from build123d import *

# Parameters (mm, degrees)
F0_W     = 72
F0_H     = 20
F0_R     = 3
F1_DEPTH = 4.5
F2_R     = 7.5
F2_R_2   = 3
F3_DEPTH = 5.5
F4_SIZE  = 5
F6_D     = 4.2


with BuildPart() as f1:
    # F0 (on Front) → F1 (new body)
    with BuildSketch(Plane.XZ):
        Rectangle(F0_W, F0_H)
        Circle(F0_R, mode=Mode.SUBTRACT)
    extrude(amount=F1_DEPTH)

    # F2 (on face) → F3 (join)
    with BuildSketch(Plane.XZ.offset(4.5)):
        Circle(F2_R)
        Circle(F2_R_2, mode=Mode.SUBTRACT)
    extrude(amount=F3_DEPTH)

    # F4
    f4_edges = [f1.edges().sort_by_distance(p)[0] for p in [
        (36, -2.25, 10),
        (36, -2.25, -10),
        (-36, -2.25, 10),
        (-36, -2.25, -10),
    ]]
    chamfer(f4_edges, length=F4_SIZE)

    # F6 (through all)
    with Locations(Plane(origin=(0, 0, 0), x_dir=(-1, 0, 0), z_dir=(0, 1, 0))):
        with Locations((-30, 0), (30, 0)):
            Hole(F6_D / 2)


solid = f1.part
For this review, take the finished solid that the model builds, in its own axes (mm). A direction names the side the tool comes from. Round coordinates to 2 decimals unless told otherwise and drop trailing zeros. Write each loop counter-clockwise with the first axis right and the second up, starting at its lowest first coordinate (ties: lowest second). Pieces come first, ordered by that corner, then holes. Notation, with made-up numbers: (-25.5, 36) - (-14.5, 36) arc R19 ccw to (-14.5, 43) - close; hole circle Ø3 at (81, 19). An arc over 180 degrees is marked (long way). Use a Markdown table: item, result.
Q1. We need section A-A (x = 30). Give the boundary of the cut face in (y, z), plus the area to 3 significant figures.
Derived:
| item | result |
|---|---|
| outline | (-4.5, -10) - (0, -10) - (0, -2.1) - (-4.5, -2.1) - close; (-4.5, 2.1) - (0, 2.1) - (0, 10) - (-4.5, 10) - close |
| area | 71.1 mm2 |
Q2. We need section C-C (y = -3.75). Give the boundary of the cut face in (x, z).
Derived:
| item | result |
|---|---|
| outline | (-36, -5) - (-31, -10) - (31, -10) - (36, -5) - (36, 5) - (31, 10) - (-31, 10) - (-36, 5) - close; hole circle Ø4.2 at (-30, 0); hole circle Ø6 at (0, 0); hole circle Ø4.2 at (30, 0) |
Q3. Clearance check with flat-ended pins moving along their axes: pin 1 (3 mm diameter, centred on x = 13.5, z = -5, fed in from -Y); pin 2 (3 mm diameter, centred on x = -0.5, z = -0.5, fed in from -Y). State where each tip first meets the part, or that it passes through.
Derived:
| item | result |
|---|---|
| pin 1 | stops at y = -4.5 |
| pin 2 | passes through |
Q4. We need section B-B (z = 0). Give the boundary of the cut face in (x, y).
Derived:
| item | result |
|---|---|
| outline | (-36, -4.5) - (-32.1, -4.5) - (-32.1, 0) - (-36, 0) - close; (-27.9, -4.5) - (-7.5, -4.5) - (-7.5, -10) - (-3, -10) - (-3, 0) - (-27.9, 0) - close; (3, -10) - (7.5, -10) - (7.5, -4.5) - (27.9, -4.5) - (27.9, 0) - (3, 0) - close; (32.1, -4.5) - (36, -4.5) - (36, 0) - (32.1, 0) - close |
Q5. Wall thickness on line 1 along X through (y, z) = (-2.5, 0.25); line 2 along Z through (x, y) = (30, -2.25); line 3 along Y through (x, z) = (5, -8.25): over which ranges is each line inside the solid? List them lowest first.
Derived:
| item | result |
|---|---|
| line 1 | x = -36 to -32.09, -27.91 to -2.99, 2.99 to 27.91, 32.09 to 36 |
| line 2 | z = -10 to -2.1, 2.1 to 10 |
| line 3 | y = -4.5 to 0 |
Q6. Machinability: for faces 1 (the cylindrical face through (-7.493, -7.212, 0.33)), 2 (the flat face through (0, -2, 10)), which of the approach directions +Z, -Z, +X, -X, +Y, -Y give a long, thin tool a straight path to every point of the face, cutting with its end or side? Answer none if there is none.
Derived:
| item | result |
|---|---|
| face 1 | -Y |
| face 2 | +Z, +X, -X, +Y, -Y |
Q7. We need section D-D (x = 0). Give the boundary of the cut face in (y, z), plus the area to 4 significant figures.
Derived:
| item | result |
|---|---|
| outline | (-10, -7.5) - (-4.5, -7.5) - (-4.5, -10) - (0, -10) - (0, -3) - (-10, -3) - close; (-10, 3) - (0, 3) - (0, 10) - (-4.5, 10) - (-4.5, 7.5) - (-10, 7.5) - close |
| area | 112.5 mm2 |
Q8. The part is to be moulded in two halves that separate along X. For faces 3 (the flat face through (-34, -2, 7)), 4 (the flat face through (33, -2, -8)), 5 (the cylindrical face through (-3, -5, 0)), say which applies: pulls with the +X half, pulls with the -X half, needs draft (parallel to the pull), parting line crosses it, or undercut.
Derived:
| item | result |
|---|---|
| face 3 | pulls with the -X half |
| face 4 | pulls with the +X half |
| face 5 | undercut |
